Verification items for the finished model (mm, model axes). Face numbers are marked on the shaded views. A direction names the side the tool comes from. Round coordinates to 2 decimals unless told otherwise and drop trailing zeros. Write each loop counter-clockwise with the first axis right and the second up, starting at its lowest first coordinate (ties: lowest second). Pieces come first, ordered by that corner, then holes. Notation, with made-up numbers: (25.5, 32.25) - (65.5, 32.25) arc R18 cw to (65.5, 50.25) - close; hole circle Ø2 at (-34, 15). An arc over 180 degrees is marked (long way). Write each question's results on one line, items separated by ' | '.
Solid Edge part; units mm, degrees
sketch "Sketch1" plane through (0, 0, 0) normal (0, 0, 1) x (1, 0, 0)
  circle A0 centre (0, 0) radius 8
extrude "Protrusion1" add sketch "Sketch1" along normal blind 4.4
sketch "Sketch2" plane through (0, 0, 0) normal (0, 0, -1) x (1, 0, 0)
  circle A0 centre (0, 0) radius 4
extrude "Protrusion2" add sketch "Sketch2" along normal blind 75.6
sketch "Sketch3" plane through (0, 0, -75.6) normal (0, 0, -1) x (1, 0, 0)
  circle A0 centre (0, 0) radius 3.9997
extrude "Cutout1" cut sketch "Sketch3" against normal blind 22 flip side to cut
chamfer "Chamfer_1" distance 0.6 angle 45 1 edges at (-3.9997, 0, -75.6)
sketch "Sketch4" plane through (0, 0, 4.4) normal (0, 0, 1) x (1, 0, 0)
  line L0 (-1.4434, 2.5) -> (1.4434, 2.5)
  line L1 (2.8868, 0) -> (1.4434, 2.5)
  line L2 (1.4434, -2.5) -> (2.8868, 0)
  line L3 (-1.4434, -2.5) -> (1.4434, -2.5)
  line L4 (-2.8868, 0) -> (-1.4434, -2.5)
  line L5 (-1.4434, 2.5) -> (-2.8868, 0)
extrude "Cutout2" cut sketch "Sketch4" against normal blind 2.9333
sketch "Sketch5" plane through (0, 0, 0) normal (0, -1, 0) x (1, 0, 0)
  line L0 (8, 4.4) -> (3.6, 0)
  line L1 (3.6, 0) -> (8, 0)
  line L2 (8, 0) -> (8, 4.4)
revolve "RevolvedCutout1" cut sketch "Sketch5" angle 360 about axis through (0, 0, 14.0017) along (0, 0, -1)
properties part number "109211"
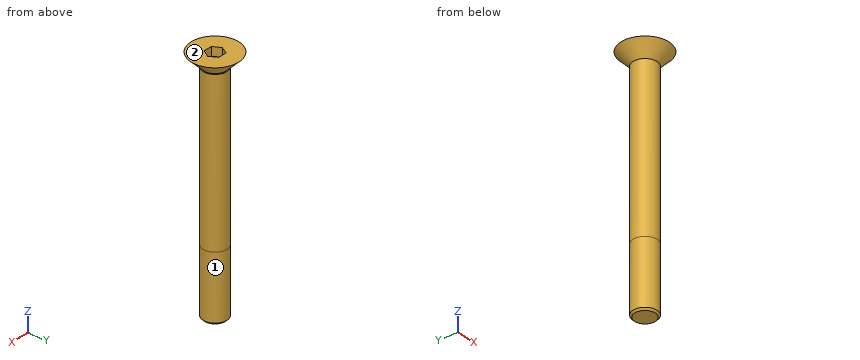
(1) Section check B-B (z = -12.5). Record the cut outline in (x, y), plus the area to 3 significant figures.
Answer:
outline: circle Ø8 at (0, 0) | area: 50.3 mm2
(2) Set-up check for the marked faces 1 and 2: record each of +Z, -Z, +X, -X, +Y, -Y from which the full face is reachable in a straight line by a thin tool's end or side.
Answer:
face 1: -Z | face 2: +Z, +X, -X, +Y, -Y
(3) Thickness scan on L1, parallel to Z at x = 1, y = -2.25; L2, parallel to X at y = 0, z = -50.5; L3, parallel to X at y = -2.75, z = -65.5. Record the ranges inside material, lowest first.
Answer:
L1: -75.6 to 1.47 | L2: -4 to 4 | L3: -2.9 to 2.9
(4) Go/stop test with flat-tipped pins: pin 1 Ø8 at (y, z) = (-0.5, -58.5) entering from +X; pin 2 Ø4 at (y, z) = (-5.5, -8) entering from +X; pin 3 Ø1.5 at (x, y) = (6, 0) entering from -Z; pin 4 Ø4 at (x, y) = (1.5, 0) entering from +Z. Record where each tip stops, or that it passes through.
Answer:
pin 1: x = 4 | pin 2: x = 1.94 | pin 3: z = 1.65 | pin 4: z = 4.4
